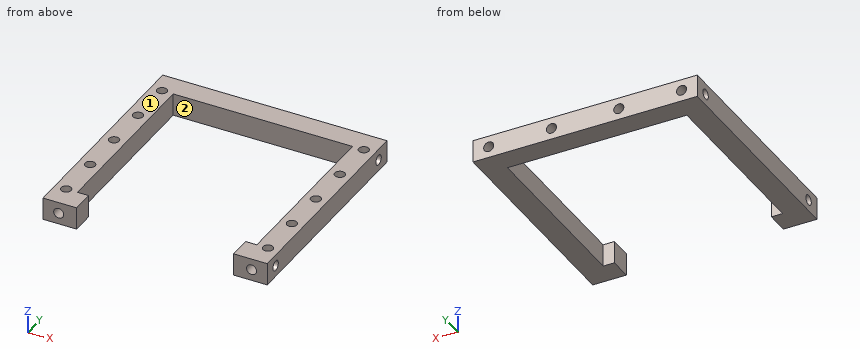
```python
from build123d import *

# Parameters (mm, degrees)
SKETCH_W              = 100
SKETCH_H              = 100
SKETCH_W_2            = 80
SKETCH_H_2            = 80
PAD_DEPTH             = 10
SKETCH002_R           = 2.25
POCKET_DEPTH          = 6
SKETCH070_R           = 2.25
POCKET044_DEPTH       = 6
POLARPATTERN_COUNT    = 4
SKETCH071_R           = 2.25
POCKET045_DEPTH       = 6
POLARPATTERN001_COUNT = 4
SKETCH072_R           = 2.25
POCKET046_DEPTH       = 6
SKETCH097_W           = 70
SKETCH097_H           = 10
POCKET060_DEPTH       = 10


with BuildPart() as part:
    # Sketch → Pad (new body)
    with BuildSketch(Plane.XY):
        Rectangle(SKETCH_W, SKETCH_H)
        Rectangle(SKETCH_W_2, SKETCH_H_2, mode=Mode.SUBTRACT)
    extrude(amount=PAD_DEPTH)

    # Sketch002 (on Face10 of Pad) → Pocket (cut)
    with BuildSketch(Plane.XY.offset(10)):
        with Locations((-45, 40)):
            Circle(SKETCH002_R)
        with Locations((-45, 20)):
            Circle(SKETCH002_R)
        with Locations((-45, 0)):
            Circle(SKETCH002_R)
        with Locations((-45, -20)):
            Circle(SKETCH002_R)
        with Locations((-45, -40)):
            Circle(SKETCH002_R)
    pocket = extrude(amount=-POCKET_DEPTH, mode=Mode.SUBTRACT)

    # Mirrored: Pocket across Sketch002 V_Axis
    add(pocket.mirror(Plane(origin=(0, 0, 10), x_dir=(0, 0, 1), z_dir=(1, 0, 0))), mode=Mode.SUBTRACT)

    # Sketch070 (on Face6 of Mirrored) → Pocket044 (cut)
    with BuildSketch(Plane.XZ.offset(50)):
        with Locations((-43, 5)):
            Circle(SKETCH070_R)
    pocket044 = extrude(amount=-POCKET044_DEPTH, mode=Mode.SUBTRACT)

    # PolarPattern: Pocket044 ×4 about axis
    polarpattern_axis = Axis((0, 0, 0), (0, 0, 1))
    for i in range(1, POLARPATTERN_COUNT):
        add(pocket044.rotate(polarpattern_axis, i * 360 / POLARPATTERN_COUNT), mode=Mode.SUBTRACT)

    # Sketch071 (on Face2 of PolarPattern) → Pocket045 (cut)
    with BuildSketch(Plane(origin=(-50, 0, 0), x_dir=(0, -1, 0), z_dir=(-1, 0, 0))):
        with Locations((43, 5)):
            Circle(SKETCH071_R)
    pocket045 = extrude(amount=-POCKET045_DEPTH, mode=Mode.SUBTRACT)

    # PolarPattern001: Pocket045 ×4 about axis
    polarpattern001_axis = Axis((0, 0, 0), (0, 0, 1))
    for i in range(1, POLARPATTERN001_COUNT):
        add(pocket045.rotate(polarpattern001_axis, i * 360 / POLARPATTERN001_COUNT), mode=Mode.SUBTRACT)

    # Sketch072 (on Face1 of PolarPattern001) → Pocket046 (cut)
    with BuildSketch(Plane(origin=(0, 50, 0), x_dir=(-1, 0, 0), z_dir=(0, 1, 0))):
        with Locations((-15, 5)):
            Circle(SKETCH072_R)
    pocket046 = extrude(amount=-POCKET046_DEPTH, mode=Mode.SUBTRACT)

    # Mirrored001: Pocket046 across Sketch072 V_Axis
    add(pocket046.mirror(Plane(origin=(0, 50, 0), x_dir=(0, 1, 0), z_dir=(-1, 0, 0))), mode=Mode.SUBTRACT)

    # Sketch097 (on Face4 of Mirrored001) → Pocket060 (cut)
    with BuildSketch(Plane.XY.offset(10)):
        with Locations((0, -45)):
            Rectangle(SKETCH097_W, SKETCH097_H)
    extrude(amount=-POCKET060_DEPTH, mode=Mode.SUBTRACT)


with BuildPart() as part_1:
    # Body placement: moved
    add(part.part.moved(Location((0, 0, 100))))


solid = part_1.part
```
For this review, take the finished solid that the model builds, in its own axes (mm). Face numbers are marked on the shaded views. Coordinates: 2 decimals unless noted, no trailing zeros. Loops run counter-clockwise (first coordinate to the right, second up) from the corner with the lowest first, then second, coordinate; pieces in that order, holes last.
1. Add section C-C, the plane z = 108.75. Count the separate pieces of the cut face and the enclosed holes in it, then the cut area to 3 significant figures.
2. Insertion check: P1, Ø1.5, axis at y = 43, z = 105, coming from the -X side; P2, Ø5, axis at x = 3, z = 103, coming from the -Y side; P3, Ø1.6, axis at x = -43, z = 104.5, coming from the -Y side. Each pin has a flat end and moves straight along its axis. Give the tip position at first contact, or say it passes through.
3. Add section A-A, the plane y = -20. Give the boundary of the cut face in (x, z).
4. Mouldability with a two-part tool opening along X and no side actions: class the marked faces 1 and 2 as +X half, -X half, draft (parallel to the pull), parting line (faces both ways), or undercut.
5. Add section B-B, the plane x = -36.5. Give the boundary of the cut face in (y, z).
6. For line 1 (Y direction, x = -45, z = 108.75); line 2 (X direction, y = 10, z = 101); line 3 (Y direction, x = -45.75, z = 105), list the stretches that pass through material, from the lowest coordinate up.
Result:
1. separate pieces: 1
1. enclosed holes: 10
1. area: 2,740 mm2
2. P1: stops at x = -44
2. P2: stops at y = 40
2. P3: stops at y = -44
3. outline: (-50, 100) - (-40, 100) - (-40, 110) - (-42.75, 110) - (-42.75, 104) - (-47.25, 104) - (-47.25, 110) - (-50, 110) - close; (40, 100) - (50, 100) - (50, 110) - (47.25, 110) - (47.25, 104) - (42.75, 104) - (42.75, 110) - (40, 110) - close
4. face 1: draft
4. face 2: undercut
5. outline: (-50, 100) - (-40, 100) - (-40, 110) - (-50, 110) - close; (40, 100) - (50, 100) - (50, 110) - (40, 110) - close
6. line 1: y = -50 to -42.25, -37.75 to -22.25, -17.75 to -2.25, 2.25 to 17.75, 22.25 to 37.75, 42.25 to 50
6. line 2: x = -50 to -40, 40 to 50
6. line 3: y = -50 to -45.25, -37.88 to -22.12, -17.88 to -2.12, 2.12 to 17.88, 22.12 to 37.88, 45.25 to 50
